Geometry check sheet. Reference: the model listing, model coordinates, mm. Face numbers are marked on the shaded views. A direction names the side the tool comes from. Give positions to 0.01 mm unless a question says otherwise; leave off trailing zeros. Loops run counter-clockwise (first coordinate to the right, second up) from the corner with the lowest first, then second, coordinate; pieces in that order, holes last.
1. Cross-section at A-A, the plane y = 12. Record the cut outline in (x, z), plus the area to 3 significant figures.
2. Tool access check on the marked faces 1 and 2. Record the directions out of +Z, -Z, +X, -X, +Y, -Y that give a thin tool (end or side, any length) a straight path to the whole face; none if there is none.
3. Release check for a two-part mould opening along X. For the marked faces 3, 4 and 5 record: +X half, -X half, draft (parallel to the pull), parting line (faces both ways), or undercut.
4. Go/stop test with a flat-tipped pin: pin 1 Ø11.5 at (x, z) = (-4, 0.5) entering from +Y. Record where the tip stops, or that it passes through.
5. Cross-section at C-C, the plane x = -3.75. Record the cut outline in (y, z).
6. Cross-section at D-D, the plane z = 3. Record the cut outline in (x, y).
7. Cross-section at B-B, the plane z = -12.95. Record the cut outline in (x, y), plus the area to 3 significant figures.
8. Material ranges on L1, parallel to Z at x = 0, y = 2.4; L2, parallel to Z at x = 2.5, y = 9.75; L3, parallel to X at y = 19, z = 5, recorded low to high.
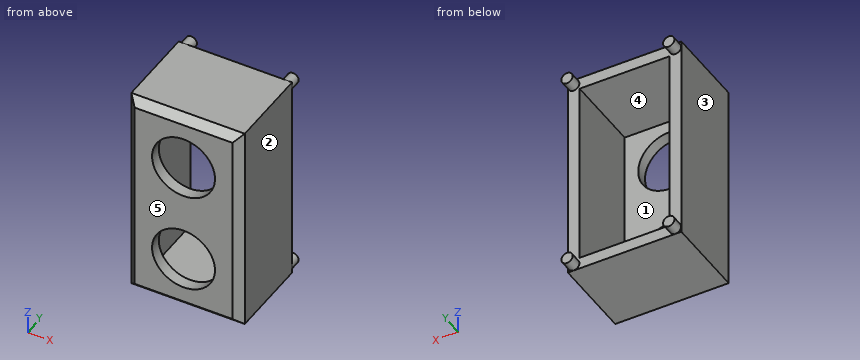
Autodesk Inventor part; units mm, degrees
ref_plane "YZ Plane" through (0, 0, 0) normal (1, 0, 0) x (0, 1, 0)
ref_plane "XZ Plane" through (0, 0, 0) normal (0, 1, 0) x (-1, 0, 0)
ref_plane "XY Plane" through (0, 0, 0) normal (0, 0, 1) x (1, 0, 0)
sketch "Sketch1" plane through (0, 0, 0) normal (0, 1, 0) x (-1, 0, 0)
  circle A0 centre (0, 12.95) radius 8.05
  circle A1 centre (0, -12.95) radius 8.05
  line L0 (14.5, 27) -> (-14.5, 27)
  line L1 (-14.5, 27) -> (-14.5, -27)
  line L2 (-14.5, -27) -> (14.5, -27)
  line L3 (14.5, -27) -> (14.5, 27)
  line L4 (14.5, 27) -> (-14.5, -27) construction
  line L5 (-14.5, 27) -> (14.5, -27) construction
  point P0 (0, 0)
  dimension "d0" = 16.1
  dimension "d1" = 16.1
  dimension "d2" = 25.9
  dimension "d3" = 29
  dimension "d4" = 54
  dimension "d5" = 14.5
  dimension "d6" = 14.5
  dimension "d7" = 14.05
  dimension "d8" = 14.05
extrude "Extrusion1" add sketch "Sketch1" along normal blind 3
sketch "Sketch12" plane through (0, 3, 0) normal (0, 1, 0) x (1, 0, 0)
  circle A0 centre (0, 12.95) radius 8.05
  circle A1 centre (0, -12.95) radius 8.05
  line L0 (-14.5, -27) -> (14.5, -27)
  line L1 (14.5, -27) -> (14.5, 27)
  line L2 (14.5, 27) -> (-14.5, 27)
  line L3 (-14.5, 27) -> (-14.5, -27)
  line L4 (14.5, -27) -> (14.5, 27)
  line L5 (-14.5, -27) -> (14.5, -27)
  line L6 (14.5, -27) -> (14.5, 27)
  line L7 (14.5, 27) -> (-14.5, 27)
  line L8 (-14.5, 27) -> (-14.5, -27)
  line L9 (-11.5, -24) -> (11.5, -24)
  line L10 (11.5, -24) -> (11.5, 24)
  line L11 (11.5, 24) -> (-11.5, 24)
  line L12 (-11.5, 24) -> (-11.5, -24)
  point P0 (0, 0)
  dimension "d85" = 3
  dimension "d86" = 3
  dimension "d87" = 3
  dimension "d88" = 3
extrude "Extrusion11" add sketch "Sketch12" along normal blind 20 contours L3 L2 L1 L0
sketch "Sketch13" plane through (0, 23, 0) normal (0, 1, 0) x (1, 0, 0)
  circle A0 centre (-13, -25.5) radius 1.45
  line L0 (-14.5, 27) -> (-14.5, -27)
  line L1 (-14.5, -27) -> (14.5, -27)
  circle A1 centre (-13, 25.5) radius 1.45
  circle A2 centre (13, -25.5) radius 1.45
  circle A3 centre (13, 25.5) radius 1.45
  point P0 (0, 0)
  dimension "d91" = 1.5
  dimension "d92" = 1.5
  dimension "d93" = 2.9
  dimension "d96" = 51
  dimension "d99" = 26
extrude "Extrusion12" add sketch "Sketch13" along normal blind 3
chamfer "Chamfer5" distance 2 angle 45 4 edges at (14.5, 0, 0) (0, 0, 27) (-14.5, 0, 0) (0, 0, -27)
sketch "Sketch2" plane through (0, 3, 0) normal (0, 1, 0) x (1, 0, 0)
  line L0 (-11.5, -24) -> (11.5, -24)
  line L1 (11.5, -24) -> (11.5, 24)
  line L2 (11.5, 24) -> (-11.5, 24)
  line L3 (-11.5, 24) -> (-11.5, -24)
  line L4 (-11.5, -24) -> (11.5, 24) construction
  line L5 (11.5, -24) -> (-11.5, 24) construction
  line L6 (14.5, -27) -> (14.5, 27)
  line L7 (-14.5, -27) -> (14.5, -27)
  line L8 (14.5, -27) -> (14.5, 27)
  line L9 (14.5, 27) -> (-14.5, 27)
  line L10 (-14.5, 27) -> (-14.5, -27)
  line L11 (-14.5, -27) -> (14.5, 27) construction
  line L12 (14.5, -27) -> (-14.5, 27) construction
  point P0 (0, 0)
  dimension "d11" = 23
  dimension "d12" = 48
sketch "Sketch3" plane through (0, 28, 0) normal (0, 1, 0) x (1, 0, 0)
  line L0 (-25.5, 27) -> (25.5, 27)
  line L1 (25.5, 27) -> (25.5, -27)
  line L2 (25.5, -27) -> (-25.5, -27)
  line L3 (-25.5, -27) -> (-25.5, 27)
  line L4 (-25.5, 27) -> (25.5, -27) construction
  line L5 (25.5, 27) -> (-25.5, -27) construction
  line L6 (14.5, -27) -> (14.5, 27)
  line L7 (-14.5, 27) -> (14.5, 27)
  line L8 (14.5, 27) -> (14.5, -27)
  line L9 (14.5, -27) -> (-14.5, -27)
  line L10 (-14.5, -27) -> (-14.5, 27)
  line L11 (-14.5, 27) -> (14.5, -27) construction
  line L12 (14.5, 27) -> (-14.5, -27) construction
  point P0 (0, 0)
  dimension "d15" = 51
sketch "Sketch4" plane through (0, 28, 0) normal (0, 1, 0) x (1, 0, 0)
  line L0 (-25.5, -27) -> (25.5, -27)
  line L1 (-25.5, 27) -> (25.5, 27)
  line L2 (25.5, 27) -> (25.5, -27)
  line L3 (25.5, -27) -> (-25.5, -27)
  line L4 (-25.5, -27) -> (-25.5, 27)
  line L5 (-25.5, 27) -> (25.5, -27) construction
  line L6 (25.5, 27) -> (-25.5, -27) construction
  line L7 (-22.5, 24) -> (22.5, 24)
  line L8 (22.5, 24) -> (22.5, -24)
  line L9 (22.5, -24) -> (-22.5, -24)
  line L10 (-22.5, -24) -> (-22.5, 24)
  line L11 (-22.5, 24) -> (22.5, -24) construction
  line L12 (22.5, 24) -> (-22.5, -24) construction
  point P0 (0, 0)
  dimension "d18" = 45
  dimension "d19" = 48
sketch "Sketch5" plane through (0, 28, 0) normal (0, 1, 0) x (1, 0, 0)
  line L0 (-11.5, 24) -> (-22.5, 24)
  line L1 (-22.5, 24) -> (-22.5, -24)
  line L2 (-22.5, -24) -> (-11.5, -24)
  line L3 (-11.5, -24) -> (-11.5, 24)
  line L4 (22.5, 24) -> (11.5, 24)
  line L5 (11.5, 24) -> (11.5, -24)
  line L6 (11.5, -24) -> (22.5, -24)
  line L7 (22.5, -24) -> (22.5, 24)
  circle A0 centre (18.5, 20) radius 1.75
  line L8 (14.5, 27) -> (14.5, -27)
  line L9 (14.5, 27) -> (25.5, 27)
  line L10 (25.5, 27) -> (25.5, -27)
  line L11 (25.5, -27) -> (14.5, -27)
  line L12 (-11.5, 24) -> (-11.5, -24)
  line L13 (-11.5, -24) -> (11.5, -24)
  line L14 (11.5, -24) -> (11.5, 24)
  line L15 (11.5, 24) -> (-11.5, 24)
  circle A1 centre (0, 12.75) radius 8.05
  circle A2 centre (0, -12.75) radius 8.05
  circle A3 centre (18.5, -20) radius 1.75
  circle A4 centre (-18.5, 20) radius 1.75
  circle A5 centre (-18.5, -20) radius 1.75
  point P0 (0, 0)
  dimension "d22" = 3.5
  dimension "d23" = 4
  dimension "d24" = 4
  dimension "d25" = 4
  dimension "d28" = 40
  dimension "d31" = 37
  dimension "d53" = 4
sketch "Sketch6" plane through (0, 25, 0) normal (0, -1, 0) x (1, 0, 0)
  line L0 (-16.5, 27) -> (-16.5, -27)
  circle A0 centre (-18.5, -20) radius 1.75
  circle A1 centre (-18.5, 20) radius 1.75
  line L1 (-16.5, 27) -> (-25.5, 27)
  line L2 (-25.5, 27) -> (-25.5, -27)
  line L3 (-25.5, -27) -> (-16.5, -27)
  line L4 (16.5, -27) -> (16.5, 27)
  circle A2 centre (18.5, -20) radius 1.75
  line L5 (16.5, -27) -> (25.5, -27)
  line L6 (25.5, -27) -> (25.5, 27)
  line L7 (25.5, 27) -> (16.5, 27)
  circle A3 centre (18.5, 20) radius 1.75
  circle A4 centre (18.5, -20) radius 3
  circle A5 centre (18.5, 20) radius 3
  circle A6 centre (-18.5, -20) radius 3
  circle A7 centre (-18.5, 20) radius 3
  point P0 (0, 0)
  dimension "d42" = 6
  dimension "d45" = 40
  dimension "d48" = 37
sketch "Sketch7" plane through (25.5, 43, -27) normal (0, 0, -1) x (-1, 0, 0)
  line L0 (40, -41) -> (11, -41)
  line L1 (40, -41) -> (40, -20)
  line L2 (42, -18) -> (40, -20)
  line L3 (51, -18) -> (42, -18)
  line L4 (51, 0) -> (51, -18)
  line L5 (0, 0) -> (51, 0)
  line L6 (0, -18) -> (0, 0)
  line L7 (9, -18) -> (0, -18)
  line L8 (11, -20) -> (9, -18)
  line L9 (11, -41) -> (11, -20)
  line L10 (0, 0) -> (51, 0)
  line L11 (18, 0) -> (33, 0)
  line L12 (33, 0) -> (33, -3)
  line L13 (33, -3) -> (18, -3)
  line L14 (18, -3) -> (18, 0)
  point P0 (25.5, -43)
  dimension "d54" = 15
  dimension "d55" = 3
  dimension "d56" = 18
  dimension "d57" = 18
  dimension "d63" = 6
equation "\"d1\" = d0"
equation "\"d7\" = d8"
equation "\"d23\" = d24"
equation "\"d25\" = d53"
equation "\"d56\" = d57"
properties part number "obudowa_baza_V2_cz1"
Result:
1. outline: (-14.5, -27) - (14.5, -27) - (14.5, 27) - (-14.5, 27) - close; hole (-11.5, -24) - (11.5, -24) - (11.5, 24) - (-11.5, 24) - close
1. area: 462 mm2
2. face 1: +Y
2. face 2: +Z, -Z, +X, +Y, -Y
3. face 3: -X half
3. face 4: undercut
3. face 5: draft
4. pin 1: stops at y = 3
5. outline: (0, -25) - (2, -27) - (23, -27) - (23, -24) - (3, -24) - (3, -20.07) - (0, -20.07) - close; (0, -5.83) - (3, -5.83) - (3, 5.83) - (0, 5.83) - close; (0, 20.07) - (3, 20.07) - (3, 24) - (23, 24) - (23, 27) - (2, 27) - (0, 25) - close
6. outline: (-14.5, 2) - (-12.5, 0) - (12.5, 0) - (14.5, 2) - (14.5, 23) - (11.5, 23) - (11.5, 3) - (-11.5, 3) - (-11.5, 23) - (-14.5, 23) - close
7. outline: (-14.5, 2) - (-12.5, 0) - (-8.05, 0) - (-8.05, 3) - (-11.5, 3) - (-11.5, 23) - (-14.5, 23) - close; (8.05, 0) - (12.5, 0) - (14.5, 2) - (14.5, 23) - (11.5, 23) - (11.5, 3) - (8.05, 3) - close
7. area: 155 mm2
8. L1: z = -27 to -21, -4.9 to 4.9, 21 to 27
8. L2: z = -27 to -24, 24 to 27
8. L3: x = -14.5 to -11.5, 11.5 to 14.5
